For this review, use the dimensioned drawing (mm, ordinates from the lowest corner) and the shaded views. A direction names the side the tool comes from. Give positions to 0.01 mm unless a question says otherwise; leave off trailing zeros. Write each loop counter-clockwise with the first axis right and the second up, starting at its lowest first coordinate (ties: lowest second). Pieces come first, ordered by that corner, then holes.
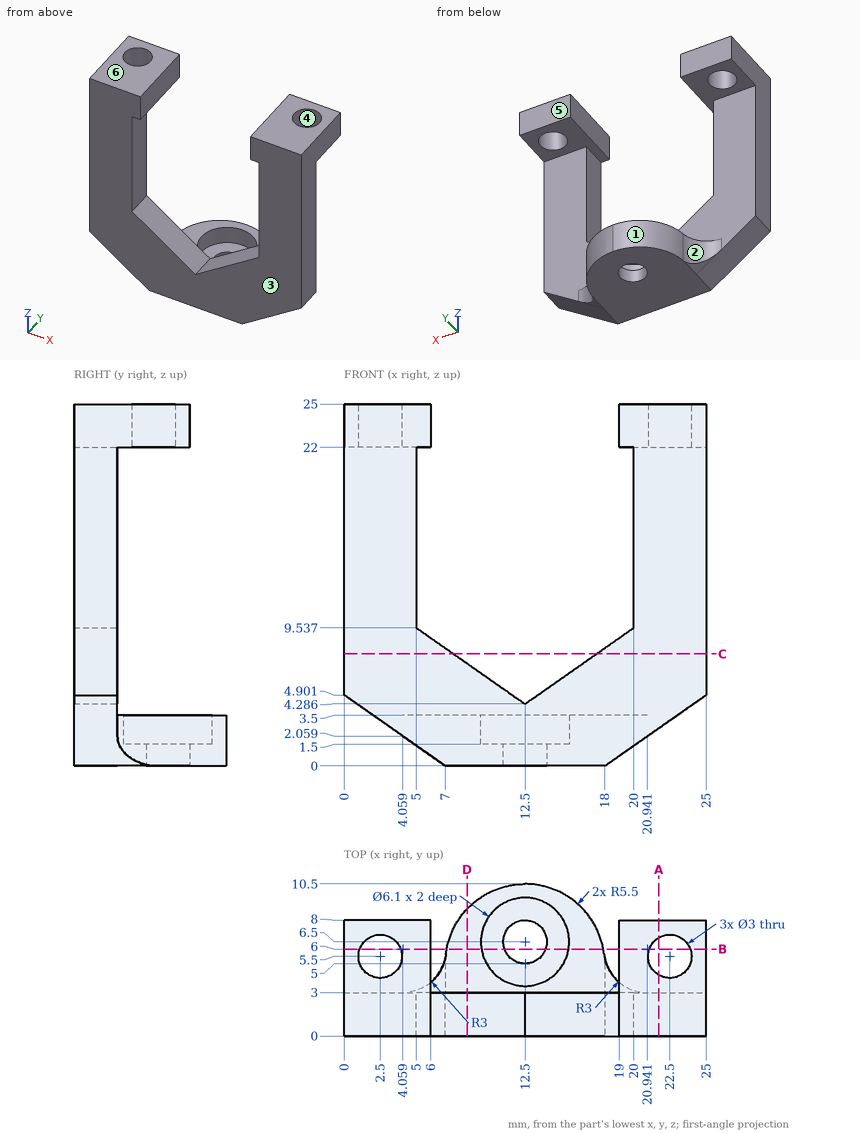
(1) Clearance check with flat-ended pins moving along their axes: pin 1 Ø6 at (x, z) = (9, 8.5) entering from +Y; pin 2 Ø2.5 at (x, z) = (21.5, 24) entering from +Y; pin 3 Ø5 at (x, y) = (12.5, 6.5) entering from +Z. State where each tip first meets the part, or that it passes through.
(2) We need section D-D (x = 8.5). Write out the cut boundary in (y, z) (1 decimal).
(3) We need section C-C (z = 7.75). Write out the cut boundary in (x, y).
(4) The part is to be moulded in two halves that separate along Y. For the marked faces 3, 4, 5 and 6, say which applies: +Y half, -Y half, draft (parallel to the pull), parting line (faces both ways), or undercut.
(5) For L1, parallel to X at y = 2, z = 22.5; L2, parallel to Y at x = 12.5, z = 0.4; L3, parallel to Y at x = 2.5, z = 23.7, list the stretches that pass through material, from the lowest coordinate up.
(6) We need section A-A (x = 21.75). Write out the cut boundary in (y, z) (1 decimal).
(7) We need section B-B (y = 6). Write out the cut boundary in (x, z) (1 decimal).
(8) Tool access review of the marked faces 1 and 2: name each direction out of +Z, -Z, +X, -X, +Y, -Y from which nothing blocks a thin tool from reaching the whole face with its end or side.
The answers:
1. pin 1: stops at y = 3
1. pin 2: stops at y = 8
1. pin 3: stops at z = 1.5
2. outline: (0, 0) - (8.8, 0) - (8.8, 3.5) - (3, 3.5) - (3, 7.1) - (0, 7.1) - close
3. outline: (0, 0) - (7.55, 0) - (7.55, 3) - (0, 3) - close; (17.45, 0) - (25, 0) - (25, 3) - (17.45, 3) - close
4. face 3: -Y half
4. face 4: undercut
4. face 5: +Y half
4. face 6: draft
5. L1: x = 0 to 6, 19 to 25
5. L2: y = 0 to 5, 8 to 10.5
5. L3: y = 0 to 4, 7 to 8
6. outline: (0, 2.6) - (3, 2.6) - (3, 22) - (4.2, 22) - (4.2, 25) - (0, 25) - close; (6.8, 22) - (8, 22) - (8, 25) - (6.8, 25) - close
7. outline: (0, 22) - (1.1, 22) - (1.1, 25) - (0, 25) - close; (3.9, 22) - (6, 22) - (6, 25) - (3.9, 25) - close; (7.1, 0) - (11.1, 0) - (11.1, 1.5) - (9.5, 1.5) - (9.5, 3.5) - (7.1, 3.5) - close; (13.9, 0) - (17.9, 0) - (17.9, 3.5) - (15.5, 3.5) - (15.5, 1.5) - (13.9, 1.5) - close; (19, 22) - (21.1, 22) - (21.1, 25) - (19, 25) - close; (23.9, 22) - (25, 22) - (25, 25) - (23.9, 25) - close
8. face 1: +Z, -Z, -X, +Y
8. face 2: -Z, -X, +Y
